from build123d import *

# Parameters (mm, degrees)
SKETCH1_R           = 40
SKETCH1_R_2         = 3.175
BOSS_EXTRUDE1_DEPTH = 7
SKETCH2_R           = 40
SKETCH2_R_2         = 4
BOSS_EXTRUDE2_DEPTH = 2.5
SKETCH3_R           = 40
SKETCH3_R_2         = 4
SKETCH3_R_3         = 3.75
BOSS_EXTRUDE3_DEPTH = 0.5


with BuildPart() as part:
    # Sketch1 → Boss-Extrude1 (new body)
    # profile 1 of 11: a face of its own
    with BuildSketch(Plane(origin=(0, 0, 0), x_dir=(0, 0, -1), z_dir=(1, 0, 0))):
        with Locations((1.5875, 0)):
            Circle(SKETCH1_R)
        with BuildLine():
            ThreePointArc((-2.741552048, 30.148588945), (-0.829517102, 34.814722887), (3.175, 31.75))
            ThreePointArc((3.175, 31.75), (3.064722887, 30.920482898), (2.741552048, 30.148588945))
            ThreePointArc((2.741552048, 30.148588945), (10.792418529, 33.215648832), (15.502933761, 26.002164676))
            ThreePointArc((15.502933761, 26.002164676), (18.82031557, 28.857349126), (21.83718176, 25.686289571))
            ThreePointArc((21.83718176, 25.686289571), (21.320571551, 23.95032047), (19.938858158, 22.779276951))
            ThreePointArc((19.938858158, 22.779276951), (28.254918529, 20.528399936), (27.8258258, 11.923797281))
            ThreePointArc((27.8258258, 11.923797281), (31.326349875, 12.77828039), (33.371044392, 9.811289571))
            ThreePointArc((33.371044392, 9.811289571), (32.187879372, 7.338797223), (29.520198147, 6.7090554))
            ThreePointArc((29.520198147, 6.7090554), (34.925, 0), (29.520198147, -6.7090554))
            ThreePointArc((29.520198147, -6.7090554), (32.187879372, -7.338797223), (33.371044392, -9.811289571))
            ThreePointArc((33.371044392, -9.811289571), (31.326349875, -12.77828039), (27.8258258, -11.923797281))
            ThreePointArc((27.8258258, -11.923797281), (28.254918529, -20.528399936), (19.938858158, -22.779276951))
            ThreePointArc((19.938858158, -22.779276951), (21.320571551, -23.95032047), (21.83718176, -25.686289571))
            ThreePointArc((21.83718176, -25.686289571), (18.82031557, -28.857349126), (15.502933761, -26.002164676))
            ThreePointArc((15.502933761, -26.002164676), (10.792418529, -33.215648832), (2.741552048, -30.148588945))
            ThreePointArc((2.741552048, -30.148588945), (3.064722887, -30.920482898), (3.175, -31.75))
            ThreePointArc((3.175, -31.75), (-0.829517102, -34.814722887), (-2.741552048, -30.148588945))
            ThreePointArc((-2.741552048, -30.148588945), (-10.792418529, -33.215648832), (-15.502933761, -26.002164676))
            ThreePointArc((-15.502933761, -26.002164676), (-20.528399936, -28.254918529), (-19.938858158, -22.779276951))
            ThreePointArc((-19.938858158, -22.779276951), (-28.254918529, -20.528399936), (-27.8258258, -11.923797281))
            ThreePointArc((-27.8258258, -11.923797281), (-33.215648832, -10.792418529), (-29.520198147, -6.7090554))
            ThreePointArc((-29.520198147, -6.7090554), (-34.925, 0), (-29.520198147, 6.7090554))
            ThreePointArc((-29.520198147, 6.7090554), (-33.215648832, 10.792418529), (-27.8258258, 11.923797281))
            ThreePointArc((-27.8258258, 11.923797281), (-28.254918529, 20.528399936), (-19.938858158, 22.779276951))
            ThreePointArc((-19.938858158, 22.779276951), (-20.528399936, 28.254918529), (-15.502933761, 26.002164676))
            ThreePointArc((-15.502933761, 26.002164676), (-10.792418529, 33.215648832), (-2.741552048, 30.148588945))
        make_face(mode=Mode.SUBTRACT)
    # profile 2 of 11: a face of its own
    with BuildSketch(Plane(origin=(0, 0, 0), x_dir=(0, 0, -1), z_dir=(1, 0, 0))):
        with Locations((18.66218176, 25.686289571)):
            Circle(SKETCH1_R_2)
    # profile 3 of 11: a face of its own
    with BuildSketch(Plane(origin=(0, 0, 0), x_dir=(0, 0, -1), z_dir=(1, 0, 0))):
        with Locations((30.196044392, 9.811289571)):
            Circle(SKETCH1_R_2)
    # profile 4 of 11: a face of its own
    with BuildSketch(Plane(origin=(0, 0, 0), x_dir=(0, 0, -1), z_dir=(1, 0, 0))):
        with Locations((30.196044392, -9.811289571)):
            Circle(SKETCH1_R_2)
    # profile 5 of 11: a face of its own
    with BuildSketch(Plane(origin=(0, 0, 0), x_dir=(0, 0, -1), z_dir=(1, 0, 0))):
        with Locations((18.66218176, -25.686289571)):
            Circle(SKETCH1_R_2)
    # profile 6 of 11: a face of its own
    with BuildSketch(Plane(origin=(0, 0, 0), x_dir=(0, 0, -1), z_dir=(1, 0, 0))):
        with Locations((0, -31.75)):
            Circle(SKETCH1_R_2)
    # profile 7 of 11: a face of its own
    with BuildSketch(Plane(origin=(0, 0, 0), x_dir=(0, 0, -1), z_dir=(1, 0, 0))):
        with Locations((-18.66218176, -25.686289571)):
            Circle(SKETCH1_R_2)
    # profile 8 of 11: a face of its own
    with BuildSketch(Plane(origin=(0, 0, 0), x_dir=(0, 0, -1), z_dir=(1, 0, 0))):
        with Locations((-30.196044392, -9.811289571)):
            Circle(SKETCH1_R_2)
    # profile 9 of 11: a face of its own
    with BuildSketch(Plane(origin=(0, 0, 0), x_dir=(0, 0, -1), z_dir=(1, 0, 0))):
        with Locations((-30.196044392, 9.811289571)):
            Circle(SKETCH1_R_2)
    # profile 10 of 11: a face of its own
    with BuildSketch(Plane(origin=(0, 0, 0), x_dir=(0, 0, -1), z_dir=(1, 0, 0))):
        with Locations((-18.66218176, 25.686289571)):
            Circle(SKETCH1_R_2)
    # profile 11 of 11: a face of its own
    with BuildSketch(Plane(origin=(0, 0, 0), x_dir=(0, 0, -1), z_dir=(1, 0, 0))):
        with Locations((0, 31.75)):
            Circle(SKETCH1_R_2)
    extrude(amount=BOSS_EXTRUDE1_DEPTH)

    # Sketch2 → Boss-Extrude2 (add)
    with BuildSketch(Plane(origin=(7, 0, 0), x_dir=(0, 0, -1), z_dir=(1, 0, 0))):
        with Locations((1.5875, 0)):
            Circle(SKETCH2_R)
        Circle(SKETCH2_R_2, mode=Mode.SUBTRACT)
    extrude(amount=BOSS_EXTRUDE2_DEPTH)

    # Sketch3 → Boss-Extrude3 (add)
    # profile 1 of 2: a face of its own
    with BuildSketch(Plane(origin=(9.5, 0, 0), x_dir=(0, 0, -1), z_dir=(1, 0, 0))):
        with Locations((1.5875, 0)):
            Circle(SKETCH3_R)
        Circle(SKETCH3_R_2, mode=Mode.SUBTRACT)
    # profile 2 of 2: a face of its own
    with BuildSketch(Plane(origin=(9.5, 0, 0), x_dir=(0, 0, -1), z_dir=(1, 0, 0))):
        Circle(SKETCH3_R_2)
        Circle(SKETCH3_R_3, mode=Mode.SUBTRACT)
    extrude(amount=BOSS_EXTRUDE3_DEPTH)

    # Sketch4 → Revolve1 (revolve)
    with BuildSketch(Plane.XY, mode=Mode.PRIVATE) as revolve1_sk:
        Polygon((10, 8.5), (10.5, 8.5), (10.5, 7.5), (15.5, 7.5), (15.5, 0), (12.325, 0), (12.325, 3.75), (10, 3.75), align=None)
    revolve(revolve1_sk.sketch.rotate(Axis((12.325, 0, 0), (1, 0, 0)), 90), axis=Axis((12.325, 0, 0), (1, 0, 0)))


solid = part.part
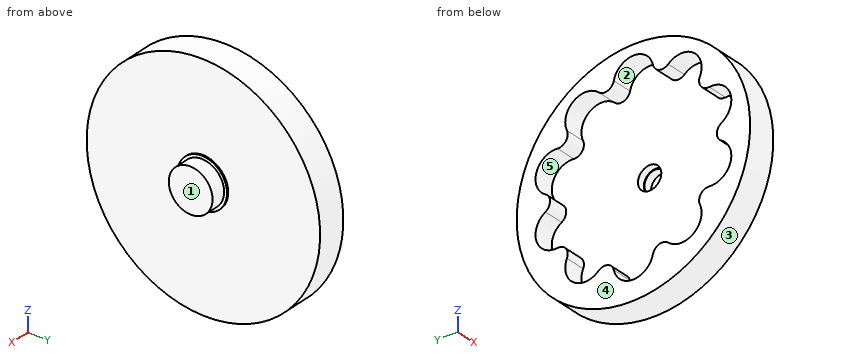
Here's how the part is built. I have some questions about the finished solid (model axes, mm). Face numbers are marked on the shaded views. A direction names the side the tool comes from. Round coordinates to 2 decimals unless told otherwise and drop trailing zeros. Write each loop counter-clockwise with the first axis right and the second up, starting at its lowest first coordinate (ties: lowest second). Pieces come first, ordered by that corner, then holes.
1. Will these pins go through, and if not, where does the flat tip stop? pin 1 Ø6.5 at (y, z) = (-1, 0.5) entering from -X; pin 2 Ø8 at (x, y) = (8.5, -11.5) entering from -Z; pin 3 Ø5 at (x, y) = (2.5, 21.5) entering from +Z.
2. For the marked faces 1 and 2, which set-ups out of +Z, -Z, +X, -X, +Y, -Y let a thin tool reach every point of the face, with its end or its side?
3. Suppose I cut it at D-D (y = -15). List the corners of the cut face in (x, z) for me, and give its area (3 significant figures).
4. Suppose I cut it at B-B (z = 22). List the corners of the cut face in (x, y) for me, and give its area (3 significant figures).
5. I need wall thicknesses on L1, parallel to Y at x = 10.7, z = 0; L2, parallel to X at y = 28, z = -30; L3, parallel to Y at x = 3, z = -6. Which ranges of each line are inside material? Lowest first, please.
6. If we mould it in two halves opening along Z, with no side actions, what happens to the marked faces 3, 4 and 5? For each: released by +Z, released by -Z, zero draft, split by the parting line, or undercut.
Answer sheet:
1. pin 1: stops at x = 7
1. pin 2: stops at z = -40.88
1. pin 3: stops at z = 33.61
2. face 1: +Z, -Z, +X, +Y, -Y
2. face 2: -X
3. outline: (0, -38.67) - (10, -38.67) - (10, 35.49) - (0, 35.49) - (0, 29.4) - (7, 29.4) - (7, -29.4) - (0, -29.4) - close
3. area: 330 mm2
4. outline: (0, -32.31) - (10, -32.31) - (10, 32.31) - (0, 32.31) - (0, 23.32) - (7, 23.32) - (7, -23.32) - (0, -23.32) - close
4. area: 320 mm2
5. L1: y = -7.5 to -3.75, 3.75 to 7.5
5. L2: x = 0 to 10
5. L3: y = -39.76 to -33.01, 33.01 to 39.76
6. face 3: split by the parting line
6. face 4: zero draft
6. face 5: undercut
